Verification items for the finished model (mm, model axes). A direction names the side the tool comes from. Round coordinates to 2 decimals unless told otherwise and drop trailing zeros. Loops run counter-clockwise (first coordinate to the right, second up) from the corner with the lowest first, then second, coordinate; pieces in that order, holes last. Notation, with made-up numbers: M 10,-24 L 55,-24 A20 ccw 55,-20 Z; hole C -12.5,15 d7. An arc over 180 degrees is marked long. Write item = value, one per line. Start each with the question number.
from build123d import *

# Parameters (mm, degrees)
EXTRUDE_THIN1_DEPTH = 14
FILLET1_R           = 7
CUT_EXTRUDE1_DEPTH  = 27.608269391
SKETCH3_R           = 2.5
CUT_EXTRUDE2_DEPTH  = 27.608269391


with BuildPart() as part:
    # Sketch1 → Extrude-Thin1 (new body)
    with BuildSketch(Plane.XY):
        Polygon((16, 0), (0, 0), (0, 16), (-1.5, 16), (-1.5, -1.5), (16, -1.5), align=None)
    extrude(amount=EXTRUDE_THIN1_DEPTH)

    # Fillet1
    fillet1_edges = [part.edges().sort_by_distance(p)[0] for p in [
        (16, -0.75, 14),
        (16, -0.75, 0),
        (-0.75, 16, 0),
        (-0.75, 16, 14),
    ]]
    fillet(fillet1_edges, radius=FILLET1_R - 0.0001)  # a hair under: the kernel refuses the full size

    # Sketch2 → Cut-Extrude1 (cut, through all)
    with BuildSketch(Plane(origin=(0, 0, 0), x_dir=(1, 0, 0), z_dir=(0, 1, 0))):
        with BuildLine():
            Line((5.90692482, -4.08603122), (10.436644309, -4.08603122))
            ThreePointArc((10.436644309, -4.08603122), (13.350613089, -7), (10.436644309, -9.91396878))
            Line((10.436644309, -9.91396878), (5.90692482, -9.91396878))
            ThreePointArc((5.90692482, -9.91396878), (2.992956041, -7), (5.90692482, -4.08603122))
        make_face()
    extrude(amount=-CUT_EXTRUDE1_DEPTH, mode=Mode.SUBTRACT)

    # Sketch3 → Cut-Extrude2 (cut, through all)
    with BuildSketch(Plane(origin=(0, 0, 0), x_dir=(0, 0, -1), z_dir=(1, 0, 0))):
        with Locations((-7, 9)):
            Circle(SKETCH3_R)
    extrude(amount=-CUT_EXTRUDE2_DEPTH, mode=Mode.SUBTRACT)


solid = part.part
1. Section check B-B, the plane x = 9.25. Enter the section's corners in (y, z).
2. Mould release check, pull along Z, two halves, no side actions. Record for faces 1 (the cylindrical face through (2.994, -0.74, 7.064)), 2 (the flat face through (-0.2, 1.8, 0)), 3 (the cylindrical face through (14, -0.7, 11.9)): pulls with the +Z half, pulls with the -Z half, needs draft (parallel to the pull), parting line crosses it, or undercut.
3. Section check A-A, the plane y = 7.75. Enter the section's corners in (x, z).
4. Gauge pin test, flat ends, axial feed: P1, Ø10, axis at x = 13, y = 7, coming from the -Z side; P2, Ø5, axis at x = 12.5, z = 3.5, coming from the +Y side; P3, Ø2, axis at y = 6.5, z = 2.5, coming from the +X side; P4, Ø6, axis at y = 9, z = 7, coming from the -X side. Record the tip position at first contact, or that the pin passes through.
5. Section check D-D, the plane z = 1. Enter the section's corners in (x, y), and give its area (3 significant figures).
6. Thickness scan on line 1 (Y direction, x = -0.6, z = 7); line 2 (X direction, y = 10.75, z = 2.5). Record the ranges inside material, lowest first.
7. Tool access check on faces 4 (the cylindrical face through (13.35, -0.74, 6.94)), 5 (the cylindrical face through (-0.8, 14, 11.9)), 6 (the flat face through (8.1, 0, 3.8)). Record the directions out of +Z, -Z, +X, -X, +Y, -Y that give a thin tool (end or side, any length) a straight path to the whole face; none if there is none.
Computed values:
q1.outline = M -1.5,0 L 0,0 L 0,4.09 L -1.5,4.09 Z; M -1.5,9.91 L 0,9.91 L 0,14 L -1.5,14 Z
q2.face_1 = undercut
q2.face_2 = pulls with the -Z half
q2.face_3 = pulls with the +Z half
q3.outline = M -1.5,0 L 0,0 L 0,4.83 L -1.5,4.83 Z; M -1.5,9.17 L 0,9.17 L 0,14 L -1.5,14 Z
q4.P1 = through
q4.P2 = 0
q4.P3 = 0
q4.P4 = -1.5
q5.outline = M -1.5,-1.5 L 12.61,-1.5 L 12.61,0 L 0,0 L 0,12.61 L -1.5,12.61 Z
q5.area = 40.1 mm2
q6.line_1 = -1.5 to 6.5, 11.5 to 16
q6.line_2 = -1.5 to 0
q7.face_4 = +Y, -Y
q7.face_5 = +Z, +X, -X, +Y
q7.face_6 = +Z, -Z, +X, +Y
